Read the model definition and answer for the solid it produces. Units are mm, in the model's axes. Face numbers are marked on the shaded views. A direction names the side the tool comes from. Round coordinates to 2 decimals unless told otherwise and drop trailing zeros. Write each loop counter-clockwise with the first axis right and the second up, starting at its lowest first coordinate (ties: lowest second). Pieces come first, ordered by that corner, then holes. Notation, with made-up numbers: (49, 36.25) -> (67, 36.25) arc R8 cw to (67, 43.25) -> close; hole circle Ø9 at (31, 7). An arc over 180 degrees is marked (long way). Return JSON: item names as keys, results as strings.
from build123d import *

# Parameters (mm, degrees)
SKETCH1_W           = 120
SKETCH1_H           = 55
BOSS_EXTRUDE1_DEPTH = 8
CUT_EXTRUDE1_REACH  = 68.485
SKETCH2_W           = 38.750815327
SKETCH2_H           = 30
SKETCH4_W           = 8
SKETCH4_H           = 10
BOSS_EXTRUDE3_DEPTH = 8
SKETCH6_W           = 20
SKETCH6_H           = 8
BOSS_EXTRUDE4_DEPTH = 8


with BuildPart() as part:
    # Sketch1 → Boss-Extrude1 (new body)
    with BuildSketch(Plane.XY):
        Rectangle(SKETCH1_W, SKETCH1_H)
    extrude(amount=BOSS_EXTRUDE1_DEPTH)

    # Sketch2 → Cut-Extrude1 (cut, up to next)
    with BuildSketch(Plane.XY.offset(8), mode=Mode.PRIVATE) as cut_extrude1_sk1:
        with Locations((-73.375407663, 0)):
            Rectangle(SKETCH2_W, SKETCH2_H)
    cut_extrude1_tool1 = extrude(cut_extrude1_sk1.sketch, amount=-CUT_EXTRUDE1_REACH, mode=Mode.PRIVATE) & part.part
    add(cut_extrude1_tool1.solids().sort_by_distance((-73.375408, 0, 8))[0], mode=Mode.SUBTRACT)

    # Sketch4 → Boss-Extrude3 (add)
    with BuildSketch(Plane(origin=(60, 0, 0), x_dir=(0, 0, -1), z_dir=(1, 0, 0))):
        with Locations((-4, 22.5)):
            Rectangle(SKETCH4_W, SKETCH4_H)
        with Locations((-4, -22.5)):
            Rectangle(SKETCH4_W, SKETCH4_H)
    boss_extrude3 = extrude(amount=BOSS_EXTRUDE3_DEPTH)

    # Sketch6 → Boss-Extrude4 (add)
    with BuildSketch(Plane.XZ.offset(27.5)):
        with Locations((-30, 4)):
            Rectangle(SKETCH6_W, SKETCH6_H)
        with Locations((30, 4)):
            Rectangle(SKETCH6_W, SKETCH6_H)
    boss_extrude4 = extrude(amount=BOSS_EXTRUDE4_DEPTH)

    # Mirror2: Boss-Extrude4 across plane
    add(boss_extrude4.mirror(Plane(origin=(0, 0, 0), x_dir=(0, 0, 1), z_dir=(0, -1, 0))))

    # Mirror3: Boss-Extrude3 across plane
    add(boss_extrude3.mirror(Plane.ZY))


solid = part.part
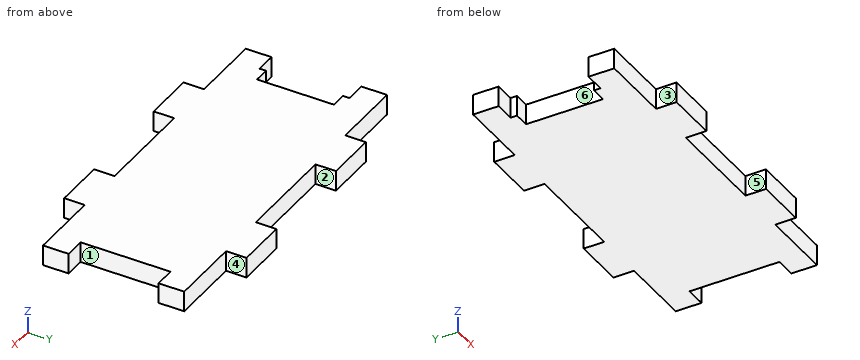
Item 1: For a pull along X with two mould halves and no side action, classify the marked faces 4, 5 and 6 as released by +X, released by -X, zero draft, split by the parting line, or undercut.
Worked answers:
{"face 4": "released by +X", "face 5": "undercut", "face 6": "released by -X"}
Item 2: Section C-C (x = -16) is taken. Give the vertices of the cut face in (y, z), then the cut area to 3 significant figures.
Worked answers:
{"outline": "(-27.5, 0) -> (27.5, 0) -> (27.5, 8) -> (-27.5, 8) -> close", "area": "440 mm2"}
Item 3: Flat-ended cylindrical pins translate along their axes: pin 1 (4 mm diameter, centred on y = -13.5, z = 4.5, fed in from +X); pin 2 (2.5 mm diameter, centred on x = -51, z = 2.5, fed in from +Y); pin 3 (1.2 mm diameter, centred on y = -16.5, z = 5.5, fed in from -X). Find the tip coordinate at first contact, or state that the pin passes through.
Worked answers:
{"pin 1": "stops at x = 60", "pin 2": "stops at y = 27.5", "pin 3": "stops at x = -60"}
Item 4: Section B-B (y = 3) is taken. Give the vertices of the cut face in (x, z).
Worked answers:
{"outline": "(-54, 0) -> (60, 0) -> (60, 8) -> (-54, 8) -> close"}
Item 5: A tool of negligible diameter and unlimited length cuts with its end or side. For the marked faces 1, 2 and 3, from which of +Z, -Z, +X, -X, +Y, -Y can it reach the whole face along a straight path? Write none if from no direction.
Worked answers:
{"face 1": "+Z, -Z, +X", "face 2": "+Z, -Z, +Y", "face 3": "+Z, -Z, -X, -Y"}
Item 6: Straight lines are drawn through the part: L1, parallel to Y at x = -47, z = 7.25; L2, parallel to X at y = 29, z = 6.5; L3, parallel to X at y = 17, z = 1.25. For each, find the intervals that lie inside material, in ascending order. Write a range as [from, to].
Worked answers:
{"L1": "y = [-27.5, 27.5]", "L2": "x = [-40, -20], [20, 40]", "L3": "x = [-60, 60]"}
